Autodesk Inventor part; units mm, degrees
ref_plane "YZ Plane" through (0, 0, 0) normal (1, 0, 0) x (0, 1, 0)
ref_plane "XZ Plane" through (0, 0, 0) normal (0, 1, 0) x (-1, 0, 0)
ref_plane "XY Plane" through (0, 0, 0) normal (0, 0, 1) x (1, 0, 0)
sketch "Sketch1" plane through (0, 0, 0) normal (0, 0, 1) x (1, 0, 0)
  line L0 (0, 0) -> (600, 0)
  line L1 (600, 0) -> (600, 600)
  line L2 (600, 600) -> (0, 600)
  line L3 (0, 600) -> (0, 0)
  circle A0 centre (300, 300) radius 50
  dimension "d0" = 600
  dimension "d1" = 600
  dimension "d5" = 100
extrude "Extrusion1" add sketch "Sketch1" along normal blind 50 contours L3 L2 L1 L0 | A0
fillet "Fillet1" radius 50 4 edges at (0, 600, 25) (600, 600, 25) (600, 0, 25) (0, 0, 25)
sketch "Sketch2" plane through (0, 0, 50) normal (0, 0, 1) x (1, 0, 0)
  circle A0 centre (300, 300) radius 50
  line L0 (50, 0) -> (550, 0)
  line L1 (550, 600) -> (50, 600)
  line L2 (600, 50) -> (600, 550)
  point P0 (0, 0)
  point P1 (300, 0)
  dimension "d6" = 100
  dimension "d7" = 300
  dimension "d8" = 300
  dimension "d9" = 300
extrude "Extrusion2" cut sketch "Sketch2" against normal through all
properties part number "Part1Grroundfinal"
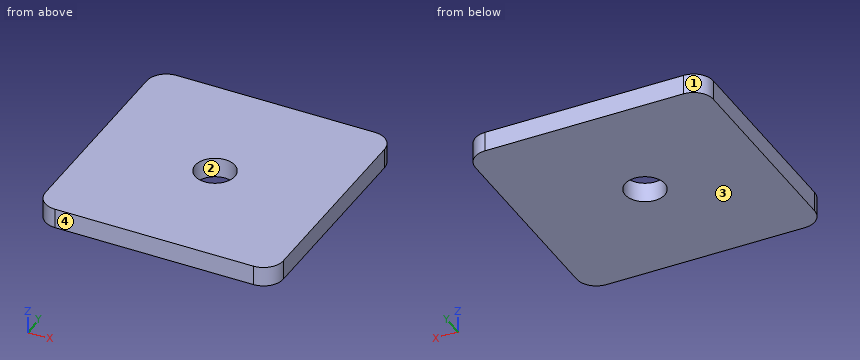
Verification items for the finished model (mm, model axes). Face numbers are marked on the shaded views. Round coordinates to 2 decimals unless told otherwise and drop trailing zeros. Write each loop counter-clockwise with the first axis right and the second up, starting at its lowest first coordinate (ties: lowest second). Pieces come first, ordered by that corner, then holes.
1. Section check A-A on x = 300. Enter the section's corners in (y, z), plus the area to 3 significant figures.
2. Draft check along Y on the marked faces 1, 2, 3 and 4. Enter one of: +Y half, -Y half, draft (parallel to the pull), parting line (faces both ways), or undercut.
3. Scan lines: L1, parallel to Y at x = 300, z = 13; L2, parallel to X at y = 344, z = 40.5; L3, parallel to Y at x = 254.5, z = 9.5. Record each from-to range of solid material in increasing order.
4. Section check C-C on z = 36. Enter the section's corners in (x, y), plus the area to 3 significant figures.
Answer:
1. outline: (0, 0) - (250, 0) - (250, 50) - (0, 50) - close; (350, 0) - (600, 0) - (600, 50) - (350, 50) - close
1. area: 25,000 mm2
2. face 1: +Y half
2. face 2: undercut
2. face 3: draft
2. face 4: -Y half
3. L1: y = 0 to 250, 350 to 600
3. L2: x = 0 to 276.25, 323.75 to 600
3. L3: y = 0 to 279.27, 320.73 to 600
4. outline: (0, 50) arc R50 ccw to (50, 0) - (550, 0) arc R50 ccw to (600, 50) - (600, 550) arc R50 ccw to (550, 600) - (50, 600) arc R50 ccw to (0, 550) - close; hole circle Ø100 at (300, 300)
4. area: 350,000 mm2
